Design review of the part built by this model. Coordinates are the model's own, in mm. A direction names the side the tool comes from. Round coordinates to 2 decimals unless told otherwise and drop trailing zeros. Loops run counter-clockwise (first coordinate to the right, second up) from the corner with the lowest first, then second, coordinate; pieces in that order, holes last. Notation, with made-up numbers: (27.5, 2) - (79.5, 2) arc R6 cw to (79.5, 6) - close; hole circle Ø4 at (1, 89.5). An arc over 180 degrees is marked (long way). Answer as CSV lines item,"result". Start each with the question number.
(1) Consider section A-A (x = 0). Give the boundary of the cut face in (y, z), and give its area (3 significant figures).
(2) For P1, Ø12, axis at x = 49, y = -41.5, coming from the +Z side; P2, Ø7, axis at x = -26.2, z = 129.5, coming from the -Y side; P3, Ø2.5, axis at x = 127, z = 88.5, coming from the +Y side, all flat-tipped, find the tip position at first contact; note any pin that passes through.
(3) For faces 1 (the flat face through (126, -78.5, 60)), 2 (the flat face through (-0.6, -78.5, -4.8)), 3 (the flat face through (-2, -41, 122)), 4 (the cylindrical face through (-0.651, -78.007, -5.043)), list the 3-axis set-ups (+Z, -Z, +X, -X, +Y, -Y) from which the entire face can be reached by the end or side of a thin tool; tool diameter is ignored.
(4) Wall thickness on L1, parallel to Z at x = 78.6, y = -0.55; L2, parallel to X at y = -15.5, z = 17.5; L3, parallel to Z at x = 28, y = -22: over which ranges is each line inside the solid? List them lowest first.
(5) Mouldability with a two-part tool opening along Y and no side actions: class faces 5 (the flat face through (126, -81, 60)), 6 (the cylindrical face through (-24.05, -0.493, 132.873)), 7 (the flat face through (-2, -1, 130)) as released by +Y, released by -Y, zero draft, split by the parting line, or undercut.
(6) Consider section C-C (x = -35). Give the boundary of the cut face in (y, z).
(7) Consider section B-B (z = 129.5). Give the boundary of the cut face in (x, y).
(8) Consider section D-D (z = 111). Give the boundary of the cut face in (x, y).
from build123d import *

# Parameters (mm, degrees)
F1_DEPTH = 122
F2_W     = 260
F2_H     = 1
F3_DEPTH = 78.5
F4_W     = 3
F4_H     = 1.5
F5_DEPTH = 1
F6_W     = 262
F6_H     = 15
F6_R     = 4
F7_DEPTH = 1
F8_R     = 5
F9_DEPTH = 1


with BuildPart() as f1:
    # F0 (on Top) → F1 (new body)
    with BuildSketch(Plane.XY):
        Polygon((-130, 0), (-131, 0), (-131, -82), (-122, -82), (-122, -81), (-130, -81), (-130, -79.5), (-122, -79.5), (-122, -78.5), (-130, -78.5), align=None)
    extrude(amount=F1_DEPTH)



with BuildPart() as f1b:
    # F0 (on Top) → F1, piece 2 (new body)
    with BuildSketch(Plane.XY):
        Polygon((131, -82), (131, 0), (130, 0), (130, -78.5), (122, -78.5), (122, -79.5), (130, -79.5), (130, -81), (122, -81), (122, -82), align=None)
    extrude(amount=F1_DEPTH)


with BuildPart() as f1_1:
    add(f1.part)

    add(f1b.part)  # F3 merges F1b
    # F2 (on Front) → F3 (join)
    with BuildSketch(Plane.XZ):
        with Locations((0, 0.5)):
            Rectangle(F2_W, F2_H)
        with Locations((0, 121.5)):
            Rectangle(F2_W, F2_H)
    extrude(amount=F3_DEPTH)

    # F4 (on face) → F5 (join)
    with BuildSketch(Plane(origin=(0, 0, 0), x_dir=(1, 0, 0), z_dir=(0, 0, -1))):
        with Locations((-128.5, 80.25)):
            Rectangle(F4_W, F4_H)
        with Locations((128.5, 80.25)):
            Rectangle(F4_W, F4_H)
    extrude(amount=-F5_DEPTH)

    # F6 (on Front) → F7 (join)
    with BuildSketch(Plane.XZ):
        with Locations((0, -7.5)):
            Rectangle(F6_W, F6_H)
        with Locations((-78.6, -7.5)):
            Circle(F6_R, mode=Mode.SUBTRACT)
        with Locations((-26.2, -7.5)):
            Circle(F6_R, mode=Mode.SUBTRACT)
        with Locations((26.2, -7.5)):
            Circle(F6_R, mode=Mode.SUBTRACT)
        with Locations((78.6, -7.5)):
            Circle(F6_R, mode=Mode.SUBTRACT)
        with Locations((0, 129.5)):
            Rectangle(F6_W, F6_H)
        with Locations((-78.6, 129.5)):
            Circle(F6_R, mode=Mode.SUBTRACT)
        with Locations((-26.2, 129.5)):
            Circle(F6_R, mode=Mode.SUBTRACT)
        with Locations((26.2, 129.5)):
            Circle(F6_R, mode=Mode.SUBTRACT)
        with Locations((78.6, 129.5)):
            Circle(F6_R, mode=Mode.SUBTRACT)
    extrude(amount=F7_DEPTH)

    # F8 (on face) → F9 (join)
    with BuildSketch(Plane.XZ.offset(78.5)):
        with BuildLine():
            Line((20, 0), (-20, 0))
            ThreePointArc((-20, 0), (0, -20), (20, 0))
        make_face()
        with Locations((0, -10)):
            Circle(F8_R, mode=Mode.SUBTRACT)
    extrude(amount=-F9_DEPTH)


solid = f1_1.part
Determined:
1,outline,"(-78.5, -20) - (-77.5, -20) - (-77.5, -15) - (-78.5, -15) - close; (-78.5, -5) - (-77.5, -5) - (-77.5, 0) - (-1, 0) - (-1, -15) - (0, -15) - (0, 1) - (-78.5, 1) - close; (-78.5, 121) - (0, 121) - (0, 137) - (-1, 137) - (-1, 122) - (-78.5, 122) - close"
1,area,"197 mm^2"
2,P1,"stops at z = 122"
2,P2,"passes through"
2,P3,"stops at y = -78.5"
3,face 1,"+Y"
3,face 2,"+Z, -Z, -Y"
3,face 3,"+Z, +X, -X, -Y"
3,face 4,"-Y"
4,L1,"z = -15 to -11.5, -3.5 to 1, 121 to 125.5, 133.5 to 137"
4,L2,"x = -131 to -130, 130 to 131"
4,L3,"z = 0 to 1, 121 to 122"
5,face 5,"undercut"
5,face 6,"zero draft"
5,face 7,"released by -Y"
6,outline,"(-78.5, 0) - (-1, 0) - (-1, -15) - (0, -15) - (0, 1) - (-78.5, 1) - close; (-78.5, 121) - (0, 121) - (0, 137) - (-1, 137) - (-1, 122) - (-78.5, 122) - close"
7,outline,"(-131, -1) - (-82.6, -1) - (-82.6, 0) - (-131, 0) - close; (-74.6, -1) - (-30.2, -1) - (-30.2, 0) - (-74.6, 0) - close; (-22.2, -1) - (22.2, -1) - (22.2, 0) - (-22.2, 0) - close; (30.2, -1) - (74.6, -1) - (74.6, 0) - (30.2, 0) - close; (82.6, -1) - (131, -1) - (131, 0) - (82.6, 0) - close"
8,outline,"(-131, -82) - (-122, -82) - (-122, -81) - (-130, -81) - (-130, -79.5) - (-122, -79.5) - (-122, -78.5) - (-130, -78.5) - (-130, 0) - (-131, 0) - close; (122, -82) - (131, -82) - (131, 0) - (130, 0) - (130, -78.5) - (122, -78.5) - (122, -79.5) - (130, -79.5) - (130, -81) - (122, -81) - close"
